Model file for the job. Use its own axes, mm. A direction names the side the tool comes from. Give positions to 0.01 mm unless a question says otherwise; leave off trailing zeros. Order: outer loops, then holes, each group sorted by start corner. A loop starts at its lowest first (then second) coordinate and runs counter-clockwise, first axis right, second up. Notation, with made-up numbers: (61, 24) -> (118, 24) arc R13 cw to (118, 37) -> close; hole circle Ø5 at (-39, 26). An arc over 180 degrees is marked (long way). Answer in a Markdown table with one row per item. Add a question column.
Autodesk Inventor part; units mm, degrees
ref_plane "YZ Plane" through (0, 0, 0) normal (1, 0, 0) x (0, 1, 0)
ref_plane "XZ Plane" through (0, 0, 0) normal (0, 1, 0) x (-1, 0, 0)
ref_plane "XY Plane" through (0, 0, 0) normal (0, 0, 1) x (1, 0, 0)
sketch "Sketch1" plane through (0, 0, 0) normal (0, 1, 0) x (-1, 0, 0)
  line L0 (-1.8331, -3.175) -> (-3.6662, 0)
  line L1 (-3.6662, 0) -> (-1.8331, 3.175)
  line L2 (-1.8331, 3.175) -> (1.8331, 3.175)
  line L3 (1.8331, 3.175) -> (3.6662, 0)
  line L4 (3.6662, 0) -> (1.8331, -3.175)
  line L5 (1.8331, -3.175) -> (-1.8331, -3.175)
  point P0 (0, 0)
  point P1 (0, 0)
  dimension "d0" = 6.35
extrude "Body" add sketch "Sketch1" along normal blind 152.4
sketch "Sketch2" plane through (0, 152.4, 0) normal (0, 1, 0) x (1, 0, 0)
  circle A0 centre (0, 0) radius 2.0955
  dimension "d3" = 4.191
extrude "Hole 2" cut sketch "Sketch2" against normal blind 12.7
sketch "Sketch3" plane through (0, 0, 0) normal (0, -1, 0) x (1, 0, 0)
  circle A0 centre (0, 0) radius 2.0955
  dimension "d6" = 4.191
extrude "Hole 1" cut sketch "Sketch3" against normal blind 12.7
chamfer "Hole 2 Chamfer 1" distance 0.127 distance2 0.1244 1 edges at (-2.0955, 152.4, 0) measured on face at (0.0842, 152.4, 2.8101)
chamfer "Hole 1 Chamfer 1" distance 0.127 distance2 0.1244 1 edges at (-2.0955, 0, 0) measured on face at (-0.0842, 0, 2.8101)
sketch "Sketch4" plane through (0, 0, 0) normal (0, 0, 1) x (1, 0, 0)
  line L0 (1.8331, 152.4) -> (-1.8331, 152.4)
  line L1 (0, 152.4) -> (-3.0353, 152.4)
  line L2 (-3.6662, 152.4) -> (-1.8331, 152.4)
  line L3 (-3.6662, 0) -> (-3.6662, 152.4)
  arc A0 (-3.0353, 152.4) -> (-3.6662, 151.765) centre (-2.2234, 150.9624) ccw
  line L4 (-3.6662, 151.765) -> (-6.3588, 154.3647)
  line L5 (-6.3588, 154.3647) -> (0, 152.4)
  line L6 (0, 152.4) -> (0, -149.536)
  point P0 (0, 0)
  dimension "d15" = 3.0353
  dimension "d16" = 1.651
  dimension "d17" = 0.635
revolve "Hole 2 Chamfer 2" cut sketch "Sketch4" angle 360 about axis through (0, 152.4, 0) along (0, -1, 0)
sketch "Sketch5" plane through (0, 0, 0) normal (0, 0, 1) x (1, 0, 0)
  line L0 (0, 0) -> (-3.0353, 0)
  line L1 (1.8331, 0) -> (-1.8331, 0)
  line L2 (-3.6662, 0) -> (-3.6662, 152.4)
  arc A0 (-3.6662, 0.635) -> (-3.0353, 0) centre (-2.2234, 1.4376) ccw
  line L3 (0, 0) -> (0, -2.1986)
  line L4 (-3.6662, 0.635) -> (-4.1154, -0.8715)
  line L5 (-4.1154, -0.8715) -> (0, 0)
  point P0 (-3.6662, 151.765)
  dimension "d19" = 3.0353
  dimension "d20" = 1.651
  dimension "d21" = 0.635
revolve "Hole 1 Chamfer 2" cut sketch "Sketch5" angle 360 about axis through (0, 0, 0) along (0, -1, 0)
chamfer "Hole 2 Chamfer 1 For Short" [suppressed]
sketch "Sketch7" plane through (0, 0, 0) normal (0, 0, 1) x (1, 0, 0)
  line L0 (0.0002, 152.4004) -> (3.0355, 152.4)
  line L1 (3.6662, 152.4) -> (1.8331, 152.4)
  line L2 (3.6662, 0.635) -> (3.6662, 152.4)
  arc A0 (3.6662, 151.765) -> (3.0355, 152.4) centre (2.2233, 150.9626) ccw
  line L3 (3.6662, 151.765) -> (4.2665, 153.3032)
  line L4 (4.2665, 153.3032) -> (0.0002, 152.4004)
  line L5 (0.0002, 154.2061) -> (0.0002, 152.4004)
  line L6 (1.8331, 152.4) -> (-1.8331, 152.4)
  point P0 (0, 0)
  dimension "d33" = 3.0353
  dimension "d34" = 1.651
  dimension "d35" = 0.635
revolve "Hole 2 Chamfer 2 For Short" [suppressed]
properties part number "Standoff .5" material "VEX Aluminum Alloy 5052-H32"
Item 1: Saw through at B-B on y = 42. List the corners of the cut face in (x, z) (3 decimals), plus the area to 3 significant figures.
Item 2: Which spindle directions (+Z, -Z, +X, -X, +Y, -Y) get a long thin tool onto all of the face, cutting with end or side? Do faces 1 (the flat face through (-2.737, 75.134, 1.61)), 2 (the cylindrical face through (2, 146.08, -0.63)). Say none if no direction does.
Item 3: Pin check, flat tip, straight feed: pin 1 Ø3.5 at (x, z) = (0, 0) entering from -Y. Stop position of the tip, or through.
Item 4: Wall check: line 1 (X direction, y = 148.25, z = 0); line 2 (Z direction, x = 0, y = 143.75) (1 decimal); line 3 (Y direction, x = -1.5, z = 1.5). Give the ranges that are in metal, low to high.
Item 5: Two-plate mould, pull along X, no slides. Class faces 3 (the flat face through (0, 75, -3.175)), 4 (the flat face through (2.737, 75.134, -1.61)), 5 (the flat face through (0, 12.7, 0)), 6 (the cylindrical face through (2, 6.32, 0.63)): pulls with the +X half, pulls with the -X half, needs draft (parallel to the pull), parting line crosses it, or undercut.
Evaluation:
| question | item | result |
|---|---|---|
| 1 | outline | (-3.666, 0) -> (-1.833, -3.175) -> (1.833, -3.175) -> (3.666, 0) -> (1.833, 3.175) -> (-1.833, 3.175) -> close |
| 1 | area | 34.9 mm2 |
| 2 | face 1 | +Z, -X, +Y, -Y |
| 2 | face 2 | +Y |
| 3 | pin 1 | stops at y = 12.7 |
| 4 | line 1 | x = -3.67 to -2.1, 2.1 to 3.67 |
| 4 | line 2 | z = -3.2 to -2.1, 2.1 to 3.2 |
| 4 | line 3 | y = 0.1 to 152.3 |
| 5 | face 3 | needs draft |
| 5 | face 4 | pulls with the +X half |
| 5 | face 5 | undercut |
| 5 | face 6 | undercut |
